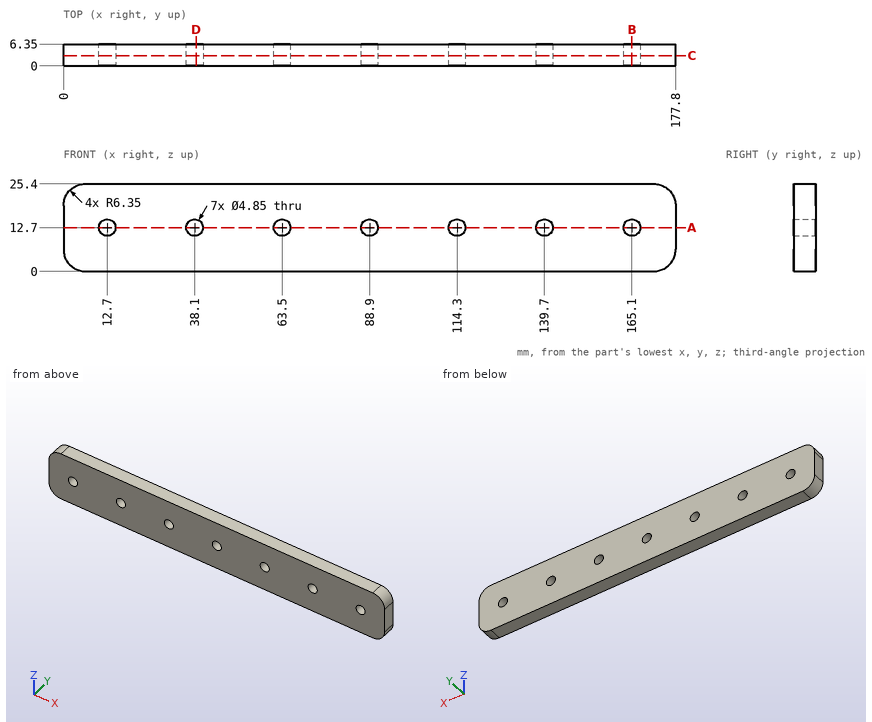
Here's the drawing with two shaded views (mm, measured from the low corner). I have some questions. Give positions to 0.01 mm unless a question says otherwise; leave off trailing zeros. Order: outer loops, then holes, each group sorted by start corner. A loop starts at its lowest first (then second) coordinate and runs counter-clockwise, first axis right, second up. Notation, with made-up numbers: (53, 44.25) -> (90, 44.25) arc R12 cw to (90, 56.25) -> close; hole circle Ø1 at (39.25, 13.5). An arc over 180 degrees is marked (long way). Use a Markdown table: item, result. Add a question column.
Item 1: Imagine slicing it at D-D on x = 38.5. Please give me the cut outline in (y, z).
Item 2: Imagine slicing it at C-C on y = 3. Please give me the cut outline in (x, z) (3 decimals), plus the area to 3 significant figures.
Item 3: I need wall thicknesses on line 1 (Z direction, x = 63.5, y = 3) (3 decimals); line 2 (Z direction, x = 137.5, y = 4); line 3 (X direction, y = 1, z = 3.25). Which ranges of each line are inside material? Lowest first, please.
Item 4: Imagine slicing it at B-B on x = 165.1. Please give me the cut outline in (y, z) (3 decimals).
Item 5: Imagine slicing it at A-A on z = 12.7. Give the number of separate pieces and of enclosed holes in the cut face, plus the area to 3 significant figures.
Item 6: Will this pin go through, and if not, where does the flat tip stop? pin 1 (3 mm diameter, centred on x = 114.3, z = 12.7, fed in from +Y).
Data:
| question | item | result |
|---|---|---|
| 1 | outline | (0, 0) -> (6.35, 0) -> (6.35, 10.31) -> (0, 10.31) -> close; (0, 15.09) -> (6.35, 15.09) -> (6.35, 25.4) -> (0, 25.4) -> close |
| 2 | outline | (0, 6.35) arc R6.35 ccw to (6.35, 0) -> (171.45, 0) arc R6.35 ccw to (177.8, 6.35) -> (177.8, 19.05) arc R6.35 ccw to (171.45, 25.4) -> (6.35, 25.4) arc R6.35 ccw to (0, 19.05) -> close; hole circle Ø4.85 at (12.7, 12.7); hole circle Ø4.85 at (38.1, 12.7); hole circle Ø4.85 at (63.5, 12.7); hole circle Ø4.85 at (88.9, 12.7); hole circle Ø4.85 at (114.3, 12.7); hole circle Ø4.85 at (139.7, 12.7); hole circle Ø4.85 at (165.1, 12.7) |
| 2 | area | 4,350 mm² |
| 3 | line 1 | z = 0 to 10.275, 15.125 to 25.4 |
| 3 | line 2 | z = 0 to 11.68, 13.72 to 25.4 |
| 3 | line 3 | x = 0.81 to 176.99 |
| 4 | outline | (0, 0) -> (6.35, 0) -> (6.35, 10.275) -> (0, 10.275) -> close; (0, 15.125) -> (6.35, 15.125) -> (6.35, 25.4) -> (0, 25.4) -> close |
| 5 | separate pieces | 8 |
| 5 | enclosed holes | 0 |
| 5 | area | 913 mm² |
| 6 | pin 1 | passes through |
